Geometry: final body of the model. Coordinates: model frame, mm. Round coordinates to 2 decimals unless told otherwise and drop trailing zeros. Write each loop counter-clockwise with the first axis right and the second up, starting at its lowest first coordinate (ties: lowest second). Pieces come first, ordered by that corner, then holes. Notation, with made-up numbers: M -38.75,-28.5 L 18.25,-28.5 A25 ccw 18.25,-12.5 Z; hole C 1,-12 d3. An arc over 180 degrees is marked long. Answer as CSV lines item,"result". Start each with the question number.
Q1. Mould query, pull axis Y, two halves, no side actions, for faces 1 (the flat face through (-8, 50, 16)), 2 (the cylindrical face through (-31.451, 17.483, 0.769)), 3 (the cylindrical face through (-45.72, 0.49, 45.49)), 4 (the flat face through (-8, -50, 16)). Classes: pulls with the +Y half, pulls with the -Y half, needs draft (parallel to the pull), parting line crosses it, or undercut.
Q2. Ray query, probe 1 along Z at (x, y) = (0, 24); probe 2 along Y at (x, z) = (34, 0.5); probe 3 along Y at (x, z) = (22, 8). Return the intervals inside material, ascending.
Q3. Section query A-A on y = 0. Output: boundary loops of the cut face in (x, z).
Q4. Section query C-C on y = -31.5. Output: boundary loops of the cut face in (x, z), and give its area (3 significant figures).
```python
from build123d import *

# Parameters (mm, degrees)
F0_W     = 100
F0_H     = 100
F1_DEPTH = 50
F2_R     = 17.5
F3_DEPTH = 100
F4_DEPTH = 100
F5_R     = 17.5
F6_DEPTH = 100
F7_R     = 17.5
F8_DEPTH = 100
F9_R     = 15


with BuildPart() as f1:
    # F0 (on Front) → F1 (new body, symmetric)
    with BuildSketch(Plane.XZ):
        Rectangle(F0_W, F0_H)
    extrude(amount=F1_DEPTH, both=True)

    # F2 (on face) → F3 (join, through all)
    with BuildSketch(Plane(origin=(-50, 0, 0), x_dir=(0, -1, 0), z_dir=(-1, 0, 0))):
        Circle(F2_R)
    extrude(amount=-F3_DEPTH)

    # F2 (on face) → F4 (cut, through all)
    with BuildSketch(Plane(origin=(-50, 0, 0), x_dir=(0, -1, 0), z_dir=(-1, 0, 0))):
        Circle(F2_R)
    extrude(amount=-F4_DEPTH, mode=Mode.SUBTRACT)

    # F5 (on face) → F6 (cut, through all)
    with BuildSketch(Plane.XZ.offset(50)):
        Circle(F5_R)
    extrude(amount=-F6_DEPTH, mode=Mode.SUBTRACT)

    # F7 (on face) → F8 (cut, through all)
    with BuildSketch(Plane(origin=(0, 0, -50), x_dir=(1, 0, 0), z_dir=(0, 0, -1))):
        Circle(F7_R)
    extrude(amount=-F8_DEPTH, mode=Mode.SUBTRACT)

    # F9
    f9_edges = [f1.edges().sort_by_distance(p)[0] for p in [
        (-50, -50, 0),
        (0, -50, 50),
        (0, -50, -50),
        (50, -50, 0),
        (50, 0, -50),
        (50, 0, 50),
        (-50, 0, 50),
        (0, 50, 50),
        (50, 50, 0),
        (-50, 50, 0),
        (0, 50, -50),
        (-50, 0, -50),
    ]]
    fillet(f9_edges, radius=F9_R)


solid = f1.part
```
Entries:
1,face 1,"pulls with the +Y half"
1,face 2,"undercut"
1,face 3,"needs draft"
1,face 4,"pulls with the -Y half"
2,probe 1,"z = -50 to -17.5, 17.5 to 50"
2,probe 2,"y = -50 to -17.49, 17.49 to 50"
2,probe 3,"y = -50 to -15.56, 15.56 to 50"
3,outline,"M -50,-35 A15 ccw -35,-50 L -17.5,-50 L -17.5,-17.5 L -50,-17.5 Z; M -50,17.5 L -17.5,17.5 L -17.5,50 L -35,50 A15 ccw -50,35 Z; M 17.5,-50 L 35,-50 A15 ccw 50,-35 L 50,-17.5 L 17.5,-17.5 Z; M 17.5,17.5 L 50,17.5 L 50,35 A15 ccw 35,50 L 17.5,50 Z"
4,outline,"M -50,-35 A15 ccw -35,-50 L 35,-50 A15 ccw 50,-35 L 50,35 A15 ccw 35,50 L -35,50 A15 ccw -50,35 Z; hole C 0,0 d35"
4,area,"8,840 mm^2"
